from build123d import *

# Parameters (mm, degrees)
F1_DEPTH = 1
F2_DEPTH = 5
F3_R     = 20.05
F3_R_2   = 19.5
F4_DEPTH = 19


with BuildPart() as f1:
    # F0 (on Top) → F1 (new body)
    with BuildSketch(Plane.XY):
        with BuildLine():
            ThreePointArc((-2.50625, 19.8927426701), (-13.2618284467, -15.0375), (20.05, 0))
            ThreePointArc((20.05, 0), (15.0333327559, 13.2665521614), (2.49375, 19.8943135327))
            ThreePointArc((2.49375, 19.8943135327), (-0.0062991589, 20.0499990105), (-2.50625, 19.8927426701))
        make_face()
    extrude(amount=F1_DEPTH)

    # F0 (on Top) → F2 (join)
    with BuildSketch(Plane.XY):
        with BuildLine():
            ThreePointArc((-2.50625, 19.8927426701), (-0.0062991589, 20.0499990105), (2.49375, 19.8943135327))
            Line((2.49375, 19.8943135327), (2.49375, 119.8927426701))
            Line((2.49375, 119.8927426701), (-2.50625, 119.8927426701))
            Line((-2.50625, 119.8927426701), (-2.50625, 19.8927426701))
        make_face()
    extrude(amount=F2_DEPTH)

    # F3 (on face) → F4 (join)
    with BuildSketch(Plane.XY.offset(1)):
        Circle(F3_R)
        Circle(F3_R_2, mode=Mode.SUBTRACT)
    extrude(amount=F4_DEPTH)


solid = f1.part
Check sheet for the modelled part. Datum: model origin and axes. Units: mm. A direction names the side the tool comes from. Round coordinates to 2 decimals unless told otherwise and drop trailing zeros. Order: outer loops, then holes, each group sorted by start corner. A loop starts at its lowest first (then second) coordinate and runs counter-clockwise, first axis right, second up.
(1) Cross-section at A-A, the plane y = 0. Enter the section's corners in (x, z), and give its area (3 significant figures).
(2) Access from +Z, -Z, +X, -X, +Y, -Y to the whole of each face (thin tool, end or side, straight path). Record for faces 4 (the flat face through (0, 71, 5)), 5 (the flat face through (2.494, 69, 2)), 6 (the flat face through (0, 119.893, 2)), 7 (the cylindrical face through (-2.539, 19.334, 10.367)), 8 (the flat face through (-2.506, 71, 2)).
(3) Cross-section at D-D, the plane x = -13. Enter the section's corners in (y, z), and give its area (3 significant figures).
(4) Cross-section at C-C, the plane x = 0. Enter the section's corners in (y, z), and give its area (3 significant figures).
(5) Go/stop test with flat-tipped pins: P1, Ø8, axis at y = 18.5, z = 11, coming from the -X side; P2, Ø4, axis at y = 72, z = 3.5, coming from the +X side; P3, Ø4, axis at x = 8, z = 4, coming from the +Y side. Record where each tip stops, or that it passes through.
(6) Cross-section at B-B, the plane z = 10.5. Enter the section's corners in (x, y), and give its area (3 significant figures).
(7) Scan lines: probe 1 along Y at (x, z) = (0, 10); probe 2 along Z at (x, y) = (-9.5, -12.5); probe 3 along Y at (x, z) = (12.5, 18.5). Record each from-to range of solid material in increasing order.
(8) Draft check along X on faces 1 (the flat face through (4.4, -19.2, 20)), 2 (the flat face through (0, 0, 1)), 3 (the cylindrical face through (-15.91, -12.2, 9.86)). Enter one of: pulls with the +X half, pulls with the -X half, needs draft (parallel to the pull), parting line crosses it, or undercut.
Check sheet entries:
1. outline: (-20.05, 0) - (20.05, 0) - (20.05, 20) - (19.5, 20) - (19.5, 1) - (-19.5, 1) - (-19.5, 20) - (-20.05, 20) - close
1. area: 61.0 mm2
2. face 4: +Z, +X, -X, +Y
2. face 5: +Z, -Z, +X, +Y
2. face 6: +Z, -Z, +X, -X, +Y
2. face 7: +Z
2. face 8: +Z, -Z, -X, +Y
3. outline: (-15.26, 0) - (15.26, 0) - (15.26, 20) - (14.53, 20) - (14.53, 1) - (-14.53, 1) - (-14.53, 20) - (-15.26, 20) - close
3. area: 58.3 mm2
4. outline: (-20.05, 0) - (119.89, 0) - (119.89, 5) - (20.05, 5) - (20.05, 20) - (19.5, 20) - (19.5, 1) - (-19.5, 1) - (-19.5, 20) - (-20.05, 20) - close
4. area: 560 mm2
5. P1: stops at x = -13.85
5. P2: stops at x = 2.49
5. P3: stops at y = 19.13
6. outline: circle Ø40.1 at (0, 0); hole circle Ø39 at (0, 0)
6. area: 68.3 mm2
7. probe 1: y = -20.05 to -19.5, 19.5 to 20.05
7. probe 2: z = 0 to 1
7. probe 3: y = -15.68 to -14.97, 14.97 to 15.68
8. face 1: needs draft
8. face 2: undercut
8. face 3: parting line crosses it
